Read the model definition and answer for the solid it produces. Units are mm, in the model's axes. A direction names the side the tool comes from. Coordinates: 2 decimals unless noted, no trailing zeros. Order: outer loops, then holes, each group sorted by start corner. A loop starts at its lowest first (then second) coordinate and runs counter-clockwise, first axis right, second up.
```python
from build123d import *

# Parameters (mm, degrees)
BOSS_EXTRUDE1_DEPTH = 50
BOSS_EXTRUDE2_DEPTH = 16.5
CUT_EXTRUDE1_DEPTH  = 16.5
CUT_EXTRUDE3_DEPTH  = 173.734095702
CUT_EXTRUDE4_DEPTH  = 3
CUT_EXTRUDE5_DEPTH  = 3
FILLET1_R           = 10


with BuildPart() as part:
    # Sketch1 → Boss-Extrude1 (new body)
    with BuildSketch(Plane.XY):
        Polygon((60, 0), (0, 0), (-95.339320844, -64.307183899), (-102.608828589, -53.529695456), (-3.974498859, 13), (60, 13), align=None)
    extrude(amount=BOSS_EXTRUDE1_DEPTH)

    # Sketch3 → Boss-Extrude2 (add, symmetric)
    with BuildSketch(Plane(origin=(-3.634753873, 5.388744222, 0), x_dir=(-0.8290375725550407, -0.5591929034707483, 0), z_dir=(0.5591929034707483, -0.8290375725550407, 0))):
        with BuildLine():
            Line((135, 0), (135, -50))
            ThreePointArc((135, -50), (115, -70), (95, -50))
            Line((95, -50), (95, 0))
            ThreePointArc((95, 0), (115, 20), (135, 0))
        make_face()
        with BuildLine():
            Line((106, -50), (106, 0))
            ThreePointArc((106, 0), (115, 9), (124, 0))
            Line((124, 0), (124, -50))
            ThreePointArc((124, -50), (115, -59), (106, -50))
        make_face(mode=Mode.SUBTRACT)
    extrude(amount=BOSS_EXTRUDE2_DEPTH, both=True)

    # Sketch3<2> → Cut-Extrude1 (cut, symmetric)
    with BuildSketch(Plane(origin=(-3.634753873, 5.388744222, 0), x_dir=(-0.8290375725550407, -0.5591929034707483, 0), z_dir=(0.5591929034707483, -0.8290375725550407, 0))):
        with BuildLine():
            Line((106, -50), (106, 0))
            ThreePointArc((106, 0), (115, 9), (124, 0))
            Line((124, 0), (124, -50))
            ThreePointArc((124, -50), (115, -59), (106, -50))
        make_face()
    extrude(amount=CUT_EXTRUDE1_DEPTH, both=True, mode=Mode.SUBTRACT)

    # Sketch5 → Cut-Extrude3 (cut, through all)
    with BuildSketch(Plane(origin=(0, 13, 0), x_dir=(1, 0, 0), z_dir=(0, 1, 0))):
        with BuildLine():
            Line((40, -37.5), (60, -37.5))
            Line((60, -37.5), (60, -12.5))
            Line((60, -12.5), (40, -12.5))
            ThreePointArc((40, -12.5), (27.5, -25), (40, -37.5))
        make_face()
    extrude(amount=-CUT_EXTRUDE3_DEPTH, mode=Mode.SUBTRACT)

    # Sketch5<3> → Cut-Extrude4 (cut)
    with BuildSketch(Plane(origin=(0, 13, 0), x_dir=(1, 0, 0), z_dir=(0, 1, 0))):
        with BuildLine():
            Line((60, -37.5), (40, -37.5))
            ThreePointArc((40, -37.5), (27.5, -25), (40, -12.5))
            Line((40, -12.5), (60, -12.5))
            ThreePointArc((60, -12.5), (72.5, -25), (60, -37.5))
        make_face()
        with BuildLine():
            Line((-3.974498859, -12.5), (1.025501141, -12.5))
            ThreePointArc((1.025501141, -12.5), (13.525501141, -25), (1.025501141, -37.5))
            Line((1.025501141, -37.5), (-3.974498859, -37.5))
            ThreePointArc((-3.974498859, -37.5), (-16.474498859, -25), (-3.974498859, -12.5))
        make_face()
    extrude(amount=-CUT_EXTRUDE4_DEPTH, mode=Mode.SUBTRACT)

    # Sketch6 → Cut-Extrude5 (cut)
    with BuildSketch(Plane(origin=(-7.269507745, 10.777488443, 0), x_dir=(0.8290375725550407, 0.5591929034707483, 0), z_dir=(-0.5591929034707483, 0.8290375725550407, 0))):
        with BuildLine():
            Line((-78.525501141, -12.5), (3.974498859, -12.5))
            ThreePointArc((3.974498859, -12.5), (16.474498859, -25), (3.974498859, -37.5))
            Line((3.974498859, -37.5), (-78.525501141, -37.5))
            ThreePointArc((-78.525501141, -37.5), (-91.025501141, -25), (-78.525501141, -12.5))
        make_face()
    extrude(amount=-CUT_EXTRUDE5_DEPTH, mode=Mode.SUBTRACT)

    # Fillet1
    fillet1_edges = [part.edges().sort_by_distance(p)[0] for p in [
        (60, 6.5, 50),
        (60, 6.5, 0),
    ]]
    fillet(fillet1_edges, radius=FILLET1_R)


solid = part.part
```
1) Straight lines are drawn through the part: line 1 (Y direction, x = 30, z = 45); line 2 (X direction, y = -56, z = 9.5); line 3 (Z direction, x = -101, y = -64.5). For each, find the intervals that lie inside material, in ascending order.
A:
line 1: y = 0 to 13
line 2: x = -124.15 to -111.8, -90.09 to -76.82
line 3: z = -19.42 to -7.61, 57.61 to 69.42
2) Which of the six approach directions +Z, -Z, +X, -X, +Y, -Y give full straight-line access (tool end or side, diameter ignored) to faces 1 (the cylindrical face through (-81.9, -41.35, 25.27)), 2 (the cylindrical face through (-99, -59, -9)), 3 (the flat face through (-45.576, -15.06, 41.317)), 4 (the flat face through (50, 7, 37.5)), 5 (the flat face through (24, 0, 25))?
A:
face 1: +Y
face 2: none
face 3: +Z, -Z, +Y
face 4: +X, +Y, -Y
face 5: +Z, -Z, +X, -Y
3) A cutting plane is placed at B-B, the plane z = 27. Determine the outline of the cut face in (x, y).
A:
outline: (-124.78, -56.42) - (-106.33, -83.78) - (-97.21, -77.63) - (-115.66, -50.27) - close; (-100.74, -40.21) - (-82.29, -67.56) - (-73.17, -61.41) - (-78.76, -53.12) - (0, 0) - (27.66, 0) - (27.66, 13) - (13.36, 13) - (13.36, 10) - (-3.06, 10) - (-80.92, -42.52) - (-82.6, -40.03) - (-86.03, -42.35) - (-91.62, -34.06) - close
4) A cutting plane is placed at D-D, the plane z = 17.5. Determine the outline of the cut face in (x, y).
A:
outline: (-124.78, -56.42) - (-106.33, -83.78) - (-97.21, -77.63) - (-115.66, -50.27) - close; (-100.74, -40.21) - (-82.29, -67.56) - (-73.17, -61.41) - (-78.76, -53.12) - (0, 0) - (30, 0) - (30, 13) - (11.03, 13) - (11.03, 10) - (-3.06, 10) - (-78.98, -41.21) - (-80.66, -38.73) - (-86.03, -42.35) - (-91.62, -34.06) - close
5) A cutting plane is placed at A-A, the plane x = 47. Determine the outline of the cut face in (y, z).
A:
outline: (0, 0) - (13, 0) - (13, 12.5) - (0, 12.5) - close; (0, 37.5) - (13, 37.5) - (13, 50) - (0, 50) - close
6) Determine the mould class of faces 6 (the flat face through (-18, -10, 50)), 7 (the flat face through (-88.785, -38.259, 25.35)), 8 (the cylindrical face through (-99, -59, 70)) for opening direction X: pulls with the +X half, pulls with the -X half, needs draft (parallel to the pull), parting line crosses it, or undercut.
A:
face 6: needs draft
face 7: undercut
face 8: parting line crosses it
7) Flat-ended cylindrical pins translate along their axes: pin 1 Ø3 at (y, z) = (-72, 39) entering from -X; pin 2 Ø6.5 at (x, y) = (50.5, 5) entering from -Z; pin 3 Ø2 at (x, z) = (-77.5, 25.5) entering from -Y; pin 4 Ø13.5 at (x, z) = (1, 31) entering from +Y. Find the tip coordinate at first contact, or state that the pin passes through.
A:
pin 1: stops at x = -115.29
pin 2: stops at z = 0
pin 3: stops at y = -65.01
pin 4: stops at y = 13
8) A cutting plane is placed at C-C, the plane y = -6. Determine the outline of the cut face in (x, z), and give its area (3 significant figures).
A:
outline: (-32.14, 0) - (-8.9, 0) - (-8.9, 50) - (-32.14, 50) - (-32.14, 37.5) - (-26.78, 37.5) - (-26.78, 12.5) - (-32.14, 12.5) - close
area: 1,030 mm2
